```python
from build123d import *

# Parameters (mm, degrees)
SKETCH2_W           = 20
SKETCH2_H           = 35
BOSS_EXTRUDE1_DEPTH = 3
SKETCH3_W           = 2
SKETCH3_H           = 35
SKETCH3_W_2         = 2.000552232
BOSS_EXTRUDE2_DEPTH = 35
SKETCH4_W           = 35
SKETCH4_H           = 2.991859995
BOSS_EXTRUDE3_DEPTH = 15
SKETCH5_W           = 35
SKETCH5_H           = 2.991859995
BOSS_EXTRUDE4_DEPTH = 15
SKETCH6_W           = 15.999447768
SKETCH6_H           = 1.992266861
BOSS_EXTRUDE5_DEPTH = 5
SKETCH8_R           = 1.45
CUT_EXTRUDE1_DEPTH  = 56.358026135
FILLET1_R           = 1
FILLET3_R           = 1


with BuildPart() as part:
    # Sketch2 → Boss-Extrude1 (new body)
    with BuildSketch(Plane(origin=(0, 0, 0), x_dir=(1, 0, 0), z_dir=(0, 1, 0))):
        with Locations((10, 2.387459807)):
            Rectangle(SKETCH2_W, SKETCH2_H)
    extrude(amount=BOSS_EXTRUDE1_DEPTH)

    # Sketch3 → Boss-Extrude2 (add)
    with BuildSketch(Plane(origin=(0, 3, 0), x_dir=(1, 0, 0), z_dir=(0, 1, 0))):
        with Locations((1, 2.387459807)):
            Rectangle(SKETCH3_W, SKETCH3_H)
        with Locations((18.999723884, 2.387459807)):
            Rectangle(SKETCH3_W_2, SKETCH3_H)
    extrude(amount=BOSS_EXTRUDE2_DEPTH)

    # Sketch4 → Boss-Extrude3 (add)
    with BuildSketch(Plane(origin=(20, 0, 0), x_dir=(0, 0, -1), z_dir=(1, 0, 0))):
        with Locations((2.387459807, 36.504070003)):
            Rectangle(SKETCH4_W, SKETCH4_H)
    extrude(amount=BOSS_EXTRUDE3_DEPTH)

    # Sketch5 → Boss-Extrude4 (add)
    with BuildSketch(Plane.ZY):
        with Locations((-2.387459807, 36.504070003)):
            Rectangle(SKETCH5_W, SKETCH5_H)
    extrude(amount=BOSS_EXTRUDE4_DEPTH)

    # Sketch6 → Boss-Extrude5 (add)
    with BuildSketch(Plane(origin=(0, 3, 0), x_dir=(1, 0, 0), z_dir=(0, 1, 0))):
        with Locations((9.999723884, 18.891326377)):
            Rectangle(SKETCH6_W, SKETCH6_H)
    extrude(amount=BOSS_EXTRUDE5_DEPTH)

    # Sketch8 → Cut-Extrude1 (cut, through all)
    with BuildSketch(Plane(origin=(0, 38, 0), x_dir=(1, 0, 0), z_dir=(0, 1, 0))):
        with Locations(Location((-6.002072166, 2.955493098, 0), (0, 0, 270))):
            Circle(SKETCH8_R)
        with Locations(Location((26.730432143, 2.955493098, 0), (0, 0, 270))):
            Circle(SKETCH8_R)
    extrude(amount=-CUT_EXTRUDE1_DEPTH, mode=Mode.SUBTRACT)

    # Fillet1
    fillet1_edges = [part.edges().sort_by_distance(p)[0] for p in [
        (2, 38, -2.387459807),
        (17.999447768, 38, -2.387459807),
        (35, 35.008140005, -2.387459807),
        (-15, 35.008140005, -2.387459807),
    ]]
    fillet(fillet1_edges, radius=FILLET1_R)

    # Fillet3
    fillet3_edges = [part.edges().sort_by_distance(p)[0] for p in [
        (9.999723884, 8, -19.887459807),
    ]]
    fillet(fillet3_edges, radius=FILLET3_R)


solid = part.part
```
Input: part model. Units: mm. Frame: model coordinates. A direction names the side the tool comes from. Round coordinates to 2 decimals unless told otherwise and drop trailing zeros. Loops run counter-clockwise (first coordinate to the right, second up) from the corner with the lowest first, then second, coordinate; pieces in that order, holes last. Notation, with made-up numbers: M -23,43.5 L -2,43.5 A26 cw -2,58.5 Z; hole C 56,30 d4. An arc over 180 degrees is marked long. Answer in a Markdown table with one row per item. Add a question column.
1. Section C-C (z = -10.5). Output: boundary loops of the cut face in (x, y).
2. Mould query, pull axis Z, two halves, no side actions, for faces 4 (the face through (0, 17, -2)), 5 (the face through (19, 22, 15.113)), 6 (the face through (27.953, 36.525, -2.176)). Classes: released by +Z, released by -Z, zero draft, split by the parting line, or undercut.
3. Contact query for flat-ended pins moving along their axis: pin 1 (1.5 mm diameter, centred on x = 11, y = 4.5, fed in from +Z); pin 2 (1.7 mm diameter, centred on x = 26.73, z = -2.96, fed in from -Y); pin 3 (1.5 mm diameter, centred on y = 5, z = -10.5, fed in from +X); pin 4 (8 mm diameter, centred on x = 7.5, z = 3.5, fed in from +Y). Output: stop coordinate, or through.
4. Section D-D (y = 4.5). Output: boundary loops of the cut face in (x, z).
5. Ray query, probe 1 along X at (y, z) = (19.5, 12.5); probe 2 along Y at (x, z) = (9.5, 13.5); probe 3 along Y at (x, z) = (20.5, -12). Return the intervals inside material, ascending.
6. Set-up query: faces 1 (the face through (10, 3, -2)), 2 (the face through (20, 17, -2)), 3 (the face through (-8, 35.008, -3)). Return all of +Z, -Z, +X, -X, +Y, -Y with unobstructed straight access to the full face (end or side cutting, diameter ignored); none if empty.
7. Section A-A (y = 32). Output: boundary loops of the cut face in (x, z), and give its area (3 significant figures).
8. Section B-B (x = 8.5). Output: boundary loops of the cut face in (y, z).
Values follow:
| question | item | result |
|---|---|---|
| 1 | outline | M -15,36.01 A1 ccw -14,35.01 L 0,35.01 L 0,0 L 20,0 L 20,35.01 L 34,35.01 A1 ccw 35,36.01 L 35,38 L 19,38 A1 ccw 18,37 L 18,3 L 2,3 L 2,37 A1 ccw 1,38 L -15,38 Z |
| 2 | face 4 | zero draft |
| 2 | face 5 | released by +Z |
| 2 | face 6 | undercut |
| 3 | pin 1 | z = -17.9 |
| 3 | pin 2 | through |
| 3 | pin 3 | x = 20 |
| 3 | pin 4 | y = 3 |
| 4 | outline | M 0,-19.89 L 20,-19.89 L 20,15.11 L 18,15.11 L 18,-17.9 L 2,-17.9 L 2,15.11 L 0,15.11 Z |
| 5 | probe 1 | 0 to 2, 18 to 20 |
| 5 | probe 2 | 0 to 3 |
| 5 | probe 3 | 35.01 to 38 |
| 6 | face 1 | +Z, +Y |
| 6 | face 2 | +Z, -Z, +X, -Y |
| 6 | face 3 | +Z, -Z, -X, -Y |
| 7 | outline | M 0,-19.89 L 2,-19.89 L 2,15.11 L 0,15.11 Z; M 18,-19.89 L 20,-19.89 L 20,15.11 L 18,15.11 Z |
| 7 | area | 140 mm^2 |
| 8 | outline | M 0,-19.89 L 7,-19.89 A1 ccw 8,-18.89 L 8,-17.9 L 3,-17.9 L 3,15.11 L 0,15.11 Z |
